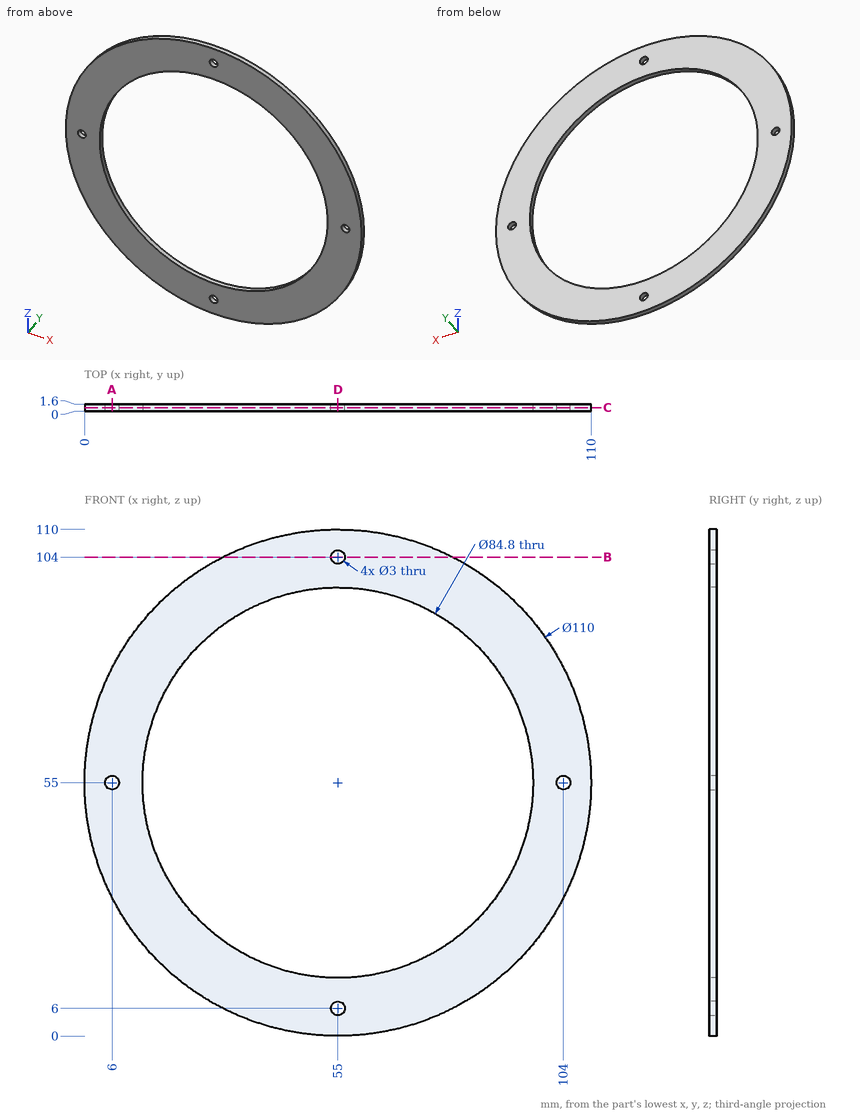
Verification items for this drawing (mm, ordinates from the low corner). Round coordinates to 2 decimals unless told otherwise and drop trailing zeros. Order: outer loops, then holes, each group sorted by start corner. A loop starts at its lowest first (then second) coordinate and runs counter-clockwise, first axis right, second up. Notation, with made-up numbers: M -9.75,-18.75 L 48.25,-18.75 A16 cw 48.25,-10.75 Z; hole C 69,43.5 d10. An arc over 180 degrees is marked long. Answer in a Markdown table with one row per item. Add a question column.
Item 1: Sectioned sample at C-C, the plane y = 0.8. Enter the section's corners in (x, z), plus the area to 3 significant figures.
Item 2: Sectioned sample at D-D, the plane x = 55. Enter the section's corners in (y, z).
Item 3: Material ranges on L1, parallel to X at y = 1.2, z = 55; L2, parallel to Z at x = 104, y = 1.25; L3, parallel to X at y = 0.5, z = 24, recorded low to high. Write a range as [from, to].
Item 4: Sectioned sample at B-B, the plane z = 104. Enter the section's corners in (x, y).
Item 5: Sectioned sample at A-A, the plane x = 6. Enter the section's corners in (y, z).
Filled in:
| question | item | result |
|---|---|---|
| 1 | outline | C 55,55 d110; hole C 6,55 d3; hole C 55,55 d84.8; hole C 55,6 d3; hole C 55,104 d3; hole C 104,55 d3 |
| 1 | area | 3,830 mm² |
| 2 | outline | M 0,0 L 1.6,0 L 1.6,4.5 L 0,4.5 Z; M 0,7.5 L 1.6,7.5 L 1.6,12.6 L 0,12.6 Z; M 0,97.4 L 1.6,97.4 L 1.6,102.5 L 0,102.5 Z; M 0,105.5 L 1.6,105.5 L 1.6,110 L 0,110 Z |
| 3 | L1 | x = [0, 4.5], [7.5, 12.6], [97.4, 102.5], [105.5, 110] |
| 3 | L2 | z = [30.02, 53.5], [56.5, 79.98] |
| 3 | L3 | x = [9.57, 26.07], [83.93, 100.43] |
| 4 | outline | M 30.02,0 L 53.5,0 L 53.5,1.6 L 30.02,1.6 Z; M 56.5,0 L 79.98,0 L 79.98,1.6 L 56.5,1.6 Z |
| 5 | outline | M 0,30.02 L 1.6,30.02 L 1.6,53.5 L 0,53.5 Z; M 0,56.5 L 1.6,56.5 L 1.6,79.98 L 0,79.98 Z |
